CAD build for the part. Positions are in the model's coordinates, mm. Face numbers are marked on the shaded views. Round coordinates to 2 decimals unless told otherwise and drop trailing zeros. Loops run counter-clockwise (first coordinate to the right, second up) from the corner with the lowest first, then second, coordinate; pieces in that order, holes last. Notation, with made-up numbers: M -23,33 L -11,33 A14 cw -11,42 Z; hole C -3.75,40 d6. An arc over 180 degrees is marked long. Put each result on its own line as item: value. Start each with the question number.
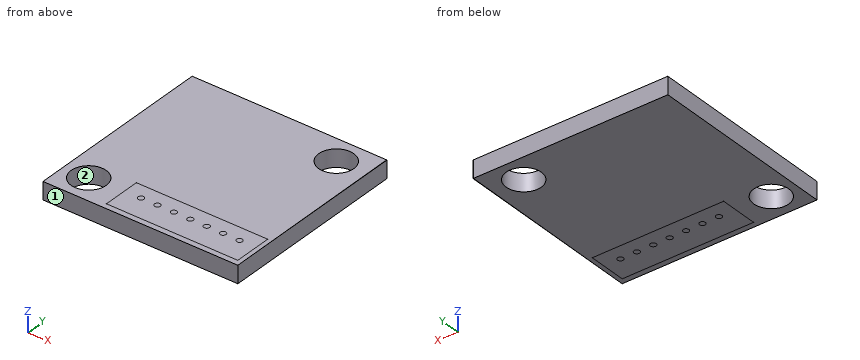
Autodesk Inventor part; units mm, degrees
ref_plane "YZ Plane" through (0, 0, 0) normal (1, 0, 0) x (0, 1, 0)
ref_plane "XZ Plane" through (0, 0, 0) normal (0, 1, 0) x (-1, 0, 0)
ref_plane "XY Plane" through (0, 0, 0) normal (0, 0, 1) x (1, 0, 0)
sketch "スケッチ1" plane through (0, 0, 0) normal (0, 0, 1) x (1, 0, 0)
  line L0 (0, 0) -> (17.8, 0)
  line L1 (17.8, 0) -> (17.76, 17.45)
  line L2 (17.76, 17.45) -> (0, 17.45)
  line L3 (0, 17.45) -> (0, 0)
  line L4 (17.399, 4.007) -> (5.399, 4.007)
  arc A0 (5.399, 4.0388) -> (5.399, 3.9753) centre (5.399, 4.007) ccw
  arc A1 (17.399, 3.9753) -> (17.399, 4.0388) centre (17.399, 4.007) ccw
  line L5 (5.399, 4.007) -> (5.399, 0.507)
  arc A2 (5.3673, 0.507) -> (5.4307, 0.507) centre (5.399, 0.507) ccw
  arc A3 (5.4307, 4.007) -> (5.3673, 4.007) centre (5.399, 4.007) ccw
  line L6 (5.399, 0.507) -> (17.399, 0.507)
  arc A4 (17.399, 0.4753) -> (17.399, 0.5388) centre (17.399, 0.5071) ccw
  arc A5 (5.399, 0.5388) -> (5.399, 0.4753) centre (5.399, 0.5071) ccw
  line L7 (17.399, 0.507) -> (17.399, 4.007)
  arc A6 (17.4307, 4.007) -> (17.3673, 4.007) centre (17.399, 4.007) ccw
  arc A7 (17.3673, 0.507) -> (17.4307, 0.507) centre (17.399, 0.507) ccw
  arc A8 (6.899, 2.8995) -> (6.899, 2.3745) centre (6.899, 2.637) ccw
  arc A9 (6.899, 2.3745) -> (6.899, 2.8995) centre (6.899, 2.637) ccw
  arc A10 (6.899, 2.8995) -> (6.899, 2.3745) centre (6.899, 2.637) ccw
  arc A11 (6.899, 2.3745) -> (6.899, 2.8995) centre (6.899, 2.637) ccw
  arc A12 (8.399, 2.8995) -> (8.399, 2.3745) centre (8.399, 2.637) ccw
  arc A13 (8.399, 2.3745) -> (8.399, 2.8995) centre (8.399, 2.637) ccw
  arc A14 (8.399, 2.8995) -> (8.399, 2.3745) centre (8.399, 2.637) ccw
  arc A15 (8.399, 2.3745) -> (8.399, 2.8995) centre (8.399, 2.637) ccw
  arc A16 (9.899, 2.8995) -> (9.899, 2.3745) centre (9.899, 2.637) ccw
  arc A17 (9.899, 2.3745) -> (9.899, 2.8995) centre (9.899, 2.637) ccw
  arc A18 (9.899, 2.8995) -> (9.899, 2.3745) centre (9.899, 2.637) ccw
  arc A19 (9.899, 2.3745) -> (9.899, 2.8995) centre (9.899, 2.637) ccw
  arc A20 (11.399, 2.8995) -> (11.399, 2.3745) centre (11.399, 2.637) ccw
  arc A21 (11.399, 2.3745) -> (11.399, 2.8995) centre (11.399, 2.637) ccw
  arc A22 (11.399, 2.8995) -> (11.399, 2.3745) centre (11.399, 2.637) ccw
  arc A23 (11.399, 2.3745) -> (11.399, 2.8995) centre (11.399, 2.637) ccw
  arc A24 (12.899, 2.8995) -> (12.899, 2.3745) centre (12.899, 2.637) ccw
  arc A25 (12.899, 2.3745) -> (12.899, 2.8995) centre (12.899, 2.637) ccw
  arc A26 (12.899, 2.8995) -> (12.899, 2.3745) centre (12.899, 2.637) ccw
  arc A27 (12.899, 2.3745) -> (12.899, 2.8995) centre (12.899, 2.637) ccw
  arc A28 (14.399, 2.8995) -> (14.399, 2.3745) centre (14.399, 2.637) ccw
  arc A29 (14.399, 2.3745) -> (14.399, 2.8995) centre (14.399, 2.637) ccw
  arc A30 (14.399, 2.8995) -> (14.399, 2.3745) centre (14.399, 2.637) ccw
  arc A31 (14.399, 2.3745) -> (14.399, 2.8995) centre (14.399, 2.637) ccw
  arc A32 (15.899, 2.8995) -> (15.899, 2.3745) centre (15.899, 2.637) ccw
  arc A33 (15.899, 2.3745) -> (15.899, 2.8995) centre (15.899, 2.637) ccw
  arc A34 (15.899, 2.8995) -> (15.899, 2.3745) centre (15.899, 2.637) ccw
  arc A35 (15.899, 2.3745) -> (15.899, 2.8995) centre (15.899, 2.637) ccw
  line L8 (0, 17.45) -> (17.8, 17.45)
  line L9 (17.8, 17.45) -> (17.8, 0)
  line L10 (17.8, 0) -> (0, 0)
  line L11 (0, 0) -> (0, 17.45)
  circle A36 centre (15.0106, 15.0866) radius 1.6
  circle A37 centre (2.3106, 2.3866) radius 1.6
  dimension "d0" = 3.2
  dimension "d1" = 3.2
  dimension "d2" = 12.7
  dimension "d3" = 12.7
extrude "押し出し1" add sketch "スケッチ1" along normal blind 1.6 contours L3 L2 L1 L0 | L1 L8 L9 | L7 L6 L5 L4 | L4 A6 A1 L7 | L4 L5 A0 A3 | A4 A7 L6 L7 | L5 L6 A2 A5 | A9 A8 | A13 A12 | A17 A16 | A21 A20 | A25 A24 | A29 A28 | A33 A32
sketch "スケッチ2" plane through (0, 0, 1.6) normal (0, 0, 1) x (1, 0, 0)
  line L0 (4.476, 11.19) -> (11.1005, 11.19) construction
  line L1 (11.1005, 11.19) -> (11.1005, 8.2657) construction
  line L2 (11.1005, 8.2657) -> (4.476, 8.2657) construction
  line L3 (4.476, 8.2657) -> (4.476, 11.19) construction
  point P0 (0, 0)
sketch "スケッチ3" plane through (0, 0, 0) normal (0, 0, -1) x (-1, 0, 0)
  line L0 (-15.9942, 10.8916) -> (2.8001, 10.8916) construction
  line L1 (2.8001, 10.8916) -> (2.8001, 7.6653) construction
  line L2 (2.8001, 7.6653) -> (-15.9942, 7.6653) construction
  line L3 (-15.9942, 7.6653) -> (-15.9942, 10.8916) construction
  line L4 (-17.4862, 3.551) -> (-6.147, 3.551)
  line L5 (-6.147, 3.551) -> (-6.147, 0.3282)
  line L6 (-6.147, 0.3282) -> (-17.4862, 0.3282)
  line L7 (-17.4862, 0.3282) -> (-17.4862, 3.551)
  point P0 (0, 0)
properties part number "Color"
(1) Cut at B-B on x = 1.5. List the corners of the cut face in (y, z).
(2) Cut at C-C on z = 1.3. List the corners of the cut face in (x, y), and give its area (3 significant figures).
(3) Drill centre lines: line 1 along X through (y, z) = (2.25, 0.5); line 2 along Y through (x, z) = (1.5, 0.4); line 3 along Y through (x, z) = (15, 0.75). Where is each one in solid material? Low to high.
(4) Cut at A-A on y = 3.25. List the corners of the cut face in (x, z), and give its area (3 significant figures).
(5) Mould opens along X. For the marked faces 1 and 2 say: +X half, -X half, draft (parallel to the pull), parting line (faces both ways), or undercut.
Taken from the geometry:
1. outline: M 0,0 L 1.01,0 L 1.01,1.6 L 0,1.6 Z; M 3.77,0 L 17.45,0 L 17.45,1.6 L 3.77,1.6 Z
2. outline: M 0,0 L 17.8,0 L 17.8,17.45 L 0,17.45 Z; hole C 2.31,2.39 d3.2; hole C 15.01,15.09 d3.2
2. area: 295 mm2
3. line 1: 0 to 0.72, 3.9 to 17.8
3. line 2: 0 to 1.01, 3.77 to 17.45
3. line 3: 0 to 13.49, 16.69 to 17.45
4. outline: M 0,0 L 0.96,0 L 0.96,1.6 L 0,1.6 Z; M 3.66,0 L 17.8,0 L 17.8,1.6 L 3.66,1.6 Z
4. area: 24.2 mm2
5. face 1: draft
5. face 2: undercut
